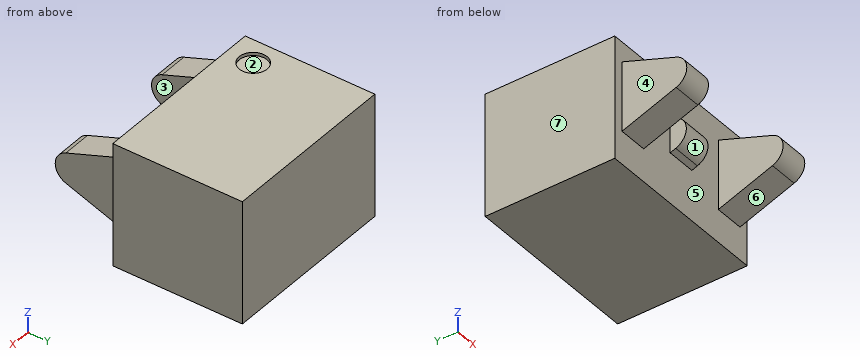
from build123d import *

# Parameters (mm, degrees)
PAD_DEPTH       = 2.75
SKETCH001_W     = 1.1
SKETCH001_H     = 5
POCKET_DEPTH    = 5
POCKET001_DEPTH = 1
SKETCH003_R     = 0.430574
POCKET002_DEPTH = 0.1


with BuildPart() as part:
    # Sketch → Pad (new body, symmetric)
    with BuildSketch(Plane.YZ):
        with BuildLine():
            Line((-2, 3.8), (2, 3.8))
            Line((2, 3.8), (2, 0))
            Line((2, 0), (-2, 0))
            Line((-2, 1.021956), (-2, 0))
            Line((-3.67101, 1.630154), (-2, 1.021956))
            ThreePointArc((-3.67101, 2.569846), (-4, 2.1), (-3.67101, 1.630154))
            Line((-3.67101, 2.569846), (-2, 3.178044))
            Line((-2, 3.8), (-2, 3.178044))
        make_face()
    extrude(amount=PAD_DEPTH, both=True)

    # Sketch001 → Pocket (cut)
    with BuildSketch(Plane.XY):
        with Locations((-3, -4.5)):
            Rectangle(SKETCH001_W, SKETCH001_H)
        with Locations((3, -4.5)):
            Rectangle(SKETCH001_W, SKETCH001_H)
        with Locations((-1, -4.5)):
            Rectangle(SKETCH001_W, SKETCH001_H)
        with Locations((1, -4.5)):
            Rectangle(SKETCH001_W, SKETCH001_H)
    extrude(amount=POCKET_DEPTH, mode=Mode.SUBTRACT)

    # Sketch002 → Pocket001 (cut, symmetric)
    with BuildSketch(Plane.YZ):
        with BuildLine():
            Line((-2, 3.803843), (-2, 2.632089))
            Line((-2.17101, 2.569846), (-2, 2.632089))
            ThreePointArc((-2.17101, 2.569846), (-2.5, 2.1), (-2.17101, 1.630154))
            Line((-2.17101, 1.630154), (-2, 1.567911))
            Line((-2, 1.567911), (-2, 0))
            Line((-2, 0), (-4.600504, 0))
            Line((-4.600504, 0), (-4.600504, 3.803843))
            Line((-4.600504, 3.803843), (-2, 3.803843))
        make_face()
    extrude(amount=POCKET001_DEPTH, both=True, mode=Mode.SUBTRACT)

    # Sketch003 (on Face5 of Pocket001) → Pocket002 (cut)
    with BuildSketch(Plane(origin=(0, 0, 3.8), x_dir=(0, -1, 0), z_dir=(0, 0, 1))):
        with Locations((1.184462, -1.98417)):
            Circle(SKETCH003_R)
    extrude(amount=-POCKET002_DEPTH, mode=Mode.SUBTRACT)


solid = part.part
Build history of the part. All positions in model axes, mm. Face numbers are marked on the shaded views. A direction names the side the tool comes from. Coordinates: 2 decimals unless noted, no trailing zeros. Order: outer loops, then holes, each group sorted by start corner. A loop starts at its lowest first (then second) coordinate and runs counter-clockwise, first axis right, second up. Notation, with made-up numbers: (18.25, 84.5) - (32.25, 84.5) arc R21 cw to (32.25, 123.5) - close; hole circle Ø8 at (26.5, -34). An arc over 180 degrees is marked (long way). Put each result on its own line as item: value.
1. Tool access for the marked faces 1, 2, 3 and 4: list every direction of +Z, -Z, +X, -X, +Y, -Y with a clear straight run to the whole face (end or side of a thin tool).
Answer sheet:
face 1: -Y
face 2: +Z
face 3: +Z, -Z, -Y
face 4: +Z, -Z, -X, -Y
2. Pull direction X, two halves, no side cores. Call the marked faces 5, 6 and 7: pulls with the +X half, pulls with the -X half, needs draft (parallel to the pull), parting line crosses it, or undercut.
Answer sheet:
face 5: undercut
face 6: needs draft
face 7: pulls with the -X half
3. Drop flat-ended pins along their axis: P1, Ø1.6, axis at y = -3, z = 2, coming from the +X side; P2, Ø1.9, axis at x = 1, z = 2.5, coming from the -Y side; P3, Ø1, axis at x = 0.5, z = 2, coming from the -Y side; P4, Ø2, axis at y = -3.5, z = 2.5, coming from the -X side. Give the stop position or say it passes through.
Answer sheet:
P1: stops at x = 2.45
P2: stops at y = -4
P3: stops at y = -2.5
P4: stops at x = -2.45
4. Saw through at D-D (x = -1.75). Write the cut outline in (y, z), and give its area (3 significant figures).
Answer sheet:
outline: (-3.67, 1.63) - (-2, 1.02) - (-2, 0) - (2, 0) - (2, 3.8) - (-0.82, 3.8) - (-0.82, 3.7) - (-1.55, 3.7) - (-1.55, 3.8) - (-2, 3.8) - (-2, 3.18) - (-3.67, 2.57) arc R0.5 ccw to start
area: 17.9 mm^2
5. Saw through at C-C (z = 0.45). Write the cut outline in (x, y).
Answer sheet:
outline: (-2.75, -2) - (2.75, -2) - (2.75, 2) - (-2.75, 2) - close
6. Saw through at A-A (y = -3.5). Write the cut outline in (x, z).
Answer sheet:
outline: (-2.45, 1.57) - (-1.55, 1.57) - (-1.55, 2.63) - (-2.45, 2.63) - close; (1.55, 1.57) - (2.45, 1.57) - (2.45, 2.63) - (1.55, 2.63) - close
7. Saw through at B-B (x = 2.2). Write the cut outline in (y, z).
Answer sheet:
outline: (-3.67, 1.63) - (-2, 1.02) - (-2, 0) - (2, 0) - (2, 3.8) - (-2, 3.8) - (-2, 3.18) - (-3.67, 2.57) arc R0.5 ccw to start
8. Probe line 1 along Y through (x, z) = (0.3, 0.2); line 2 along X through (y, z) = (-2.15, 1.25); line 3 along Y through (x, z) = (-0.1, 1.95). List the from-to ranges inside material, lowest first. Write a range as [from, to].
Answer sheet:
line 1: y = [-2, 2]
line 2: x = [-2.45, -1.55], [1.55, 2.45]
line 3: y = [-2.48, 2]
